```python
from build123d import *

# Parameters (mm, degrees)
BOSS_EXTRUDE1_DEPTH = 10
BOSS_EXTRUDE2_DEPTH = 10
SKETCH5_R           = 5
CUT_EXTRUDE1_DEPTH  = 42.419846722
FILLET1_R           = 1
FILLET2_R           = 1
FILLET3_R           = 3


with BuildPart() as part:
    # Sketch2 → Boss-Extrude1 (new body)
    with BuildSketch(Plane.XY):
        Polygon((-10, 0), (0, 0), (0, 7), (-6.25480432, 7), (-10, 1.709943763), align=None)
        Polygon((0, 0), (10, 0), (10, 1.709943763), (6.25480432, 7), (0, 7), align=None)
    extrude(amount=BOSS_EXTRUDE1_DEPTH)

    # Sketch4 → Boss-Extrude2 (add)
    with BuildSketch(Plane.XY):
        Polygon((0, 0), (-3.8, 0), (-3.8, -4.8), (-26.973388784, -4.8), (-26.973388784, -29.8), (0, -29.8), align=None)
        Polygon((3.8, 0), (0, 0), (0, -29.8), (26.973388784, -29.8), (26.973388784, -4.8), (3.8, -4.8), align=None)
    extrude(amount=BOSS_EXTRUDE2_DEPTH)

    # Sketch5 → Cut-Extrude1 (cut, through all)
    with BuildSketch(Plane.XY):
        with Locations((-19.973388784, -21.288554557)):
            Circle(SKETCH5_R)
        with Locations(Location((19.973388784, -21.288554557, 0), (0, 0, 180))):
            Circle(SKETCH5_R)
    extrude(amount=CUT_EXTRUDE1_DEPTH, mode=Mode.SUBTRACT)

    # Fillet1
    fillet1_edges = [part.edges().sort_by_distance(p)[0] for p in [
        (-10, 0, 5),
        (-10, 1.709943763, 5),
        (-6.25480432, 7, 5),
        (6.25480432, 7, 5),
        (10, 1.709943763, 5),
        (10, 0, 5),
    ]]
    fillet(fillet1_edges, radius=FILLET1_R)

    # Fillet2
    fillet2_edges = [part.edges().sort_by_distance(p)[0] for p in [
        (3.8, -4.8, 5),
        (3.8, 0, 5),
        (-3.8, 0, 5),
        (-3.8, -4.8, 5),
    ]]
    fillet(fillet2_edges, radius=FILLET2_R)

    # Fillet3
    fillet3_edges = [part.edges().sort_by_distance(p)[0] for p in [
        (-26.973388784, -29.8, 5),
        (26.973388784, -29.8, 5),
        (26.973388784, -4.8, 5),
        (-26.973388784, -4.8, 5),
    ]]
    fillet(fillet3_edges, radius=FILLET3_R)


solid = part.part
```
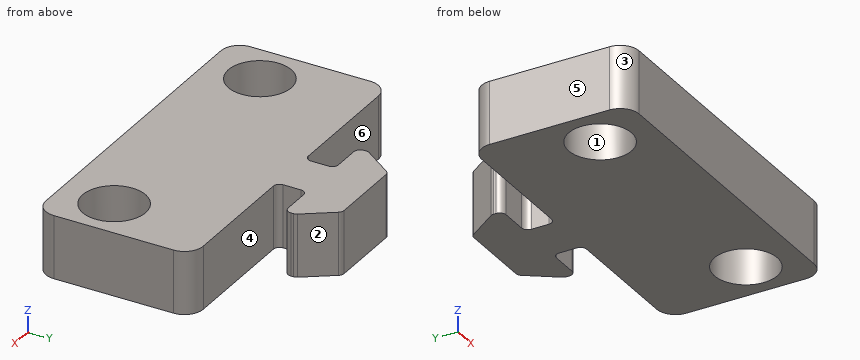
Input: part model. Units: mm. Frame: model coordinates. Face numbers are marked on the shaded views. A direction names the side the tool comes from. Coordinates: 2 decimals unless noted, no trailing zeros. Write each loop counter-clockwise with the first axis right and the second up, starting at its lowest first coordinate (ties: lowest second). Pieces come first, ordered by that corner, then holes. Notation, with made-up numbers: (-38, 82) - (-31, 82) arc R20 ccw to (-31, 89) - close; hole circle Ø7 at (38.25, 21.5). An arc over 180 degrees is marked (long way). Put each result on its own line as item: value. Start each with the question number.
1) Cut plane D-D (x = 22). Return the cut outline in (y, z).
2) Reachability of the marked faces 4, 5 and 6 from +Z, -Z, +X, -X, +Y, -Y: full face, straight path, thin tool, end or side. Return the list, or none.
3) Mould query, pull axis X, two halves, no side actions, for the marked faces 1, 2 and 3. Classes: pulls with the +X half, pulls with the -X half, needs draft (parallel to the pull), parting line crosses it, or undercut.
4) Cut plane B-B (x = -8). Return the cut outline in (y, z).
5) Cut plane A-A (y = -22). Return the cut outline in (x, z).
6) Cut plane C-C (z = 9). State how many separate pieces and enclosed holes the cut face has, plus the area to 3 significant figures.
7) Contact query for flat-ended pins moving along their axis: pin 1 (6 mm diameter, centred on x = 11.5, z = 5, fed in from +Y); pin 2 (2 mm diameter, centred on y = -2, z = 5, fed in from -X); pin 3 (1.5 mm diameter, centred on x = 11, z = 5, fed in from +Y). Output: stop coordinate, or through.
8) Ray query, L1, parallel to Y at x = -5, z = 5.5; L2, parallel to X at y = -20.5, z = 2.75; L3, parallel to X at y = -1.5, z = 9.5. Return the intervals inside material, ascending.
Resolved:
1. outline: (-29.8, 0) - (-25.86, 0) - (-25.86, 10) - (-29.8, 10) - close; (-16.72, 0) - (-4.8, 0) - (-4.8, 10) - (-16.72, 10) - close
2. face 4: +Z, -Z, +X
2. face 5: +Z, -Z, -X, +Y, -Y
2. face 6: +Z, -Z, -X
3. face 1: undercut
3. face 2: pulls with the +X half
3. face 3: pulls with the -X half
4. outline: (-29.8, 0) - (-4.8, 0) - (-4.8, 10) - (-29.8, 10) - close; (0, 0) - (4.53, 0) - (4.53, 10) - (0, 10) - close
5. outline: (-26.97, 0) - (-24.92, 0) - (-24.92, 10) - (-26.97, 10) - close; (-15.02, 0) - (15.02, 0) - (15.02, 10) - (-15.02, 10) - close; (24.92, 0) - (26.97, 0) - (26.97, 10) - (24.92, 10) - close
6. separate pieces: 1
6. enclosed holes: 2
6. area: 1,340 mm2
7. pin 1: stops at y = 3.83
7. pin 2: stops at x = -3.8
7. pin 3: stops at y = -4.8
8. L1: y = -29.8 to -4.8, 0 to 7
8. L2: x = -26.97 to -24.91, -15.04 to 15.04, 24.91 to 26.97
8. L3: x = -3.8 to 3.8
